from build123d import *

# Parameters (mm, degrees)
SKETCH1_R           = 2.5
BOSS_EXTRUDE1_DEPTH = 3
FILLET1_R           = 10
FILLET2_R           = 1
SKETCH2_R           = 1
CUT_EXTRUDE1_DEPTH  = 5


with BuildPart() as part:
    # Sketch1 → Boss-Extrude1 (new body)
    with BuildSketch(Plane.XY):
        with BuildLine():
            Line((-15.775199063, 25.595763214), (7.5, 42.17358061))
            Line((7.5, 42.17358061), (7.5, 47.084472248))
            Line((7.5, 47.084472248), (-21.353827366, 26.533263214))
            Line((-21.353827366, 26.533263214), (-10.092955814, 2.19356054))
            ThreePointArc((-10.092955814, 2.19356054), (-10.003238503, 2.060792281), (-9.876128914, 1.963223028))
            Line((-9.876128914, 1.963223028), (-7.240482475, 0.850547008))
            ThreePointArc((-7.240482475, 0.850547008), (-6.935224137, 0.406591519), (-7.210200963, -0.056730047))
            Line((-7.210200963, -0.056730047), (-9.9765648, -1.448728989))
            ThreePointArc((-9.9765648, -1.448728989), (-10.241411893, -1.996858986), (-9.780506444, -2.394548117))
            Line((-9.780506444, -2.394548117), (-6.921562347, -2.289102741))
            ThreePointArc((-6.921562347, -2.289102741), (-6.457280642, -2.56245531), (-6.510686125, -3.098577481))
            Line((-6.510686125, -3.098577481), (-8.429579039, -5.529272837))
            ThreePointArc((-8.429579039, -5.529272837), (-8.437962276, -6.137976541), (-7.852169389, -6.303618237))
            Line((-7.852169389, -6.303618237), (-5.305649232, -4.999810287))
            ThreePointArc((-5.305649232, -4.999810287), (-4.76934332, -5.051337921), (-4.591170105, -5.559799752))
            Line((-4.591170105, -5.559799752), (-5.303021449, -8.57371707))
            ThreePointArc((-5.303021449, -8.57371707), (-5.053369941, -9.128932885), (-4.45245808, -9.031488473))
            Line((-4.45245808, -9.031488473), (-2.695540082, -6.773631253))
            ThreePointArc((-2.695540082, -6.773631253), (-2.187705338, -6.593678477), (-1.811340311, -6.979202139))
            Line((-1.811340311, -6.979202139), (-1.182760229, -10.011580251))
            ThreePointArc((-1.182760229, -10.011580251), (-0.721854781, -10.409269381), (-0.21842547, -10.066998426))
            Line((-0.21842547, -10.066998426), (0.419671299, -7.278179214))
            ThreePointArc((0.419671299, -7.278179214), (0.803874553, -6.900466376), (1.307906448, -7.09081074))
            Line((1.307906448, -7.09081074), (3.159131837, -9.573429214))
            ThreePointArc((3.159131837, -9.573429214), (3.744924723, -9.73907091), (4.056536671, -9.216109658))
            Line((4.056536671, -9.216109658), (3.456242815, -6.418909742))
            ThreePointArc((3.456242815, -6.418909742), (3.644820872, -5.914214344), (4.182071907, -5.87371184))
            Line((4.182071907, -5.87371184), (6.909051797, -7.34136664))
            ThreePointArc((6.909051797, -7.34136664), (7.509963658, -7.243922228), (7.571367017, -6.638265473))
            Line((7.571367017, -6.638265473), (5.845168255, -4.356836553))
            ThreePointArc((5.845168255, -4.356836553), (5.802784524, -3.819730653), (6.272582224, -3.55597082))
            Line((6.272582224, -3.55597082), (9.364323053, -3.733646292))
            ThreePointArc((9.364323053, -3.733646292), (9.867752363, -3.391375337), (9.667441101, -2.816513723))
            Line((9.667441101, -2.816513723), (7.138800197, -1.478360048))
            ThreePointArc((7.138800197, -1.478360048), (6.87339673, -1.009488927), (7.187708321, -0.571896249))
            Line((7.187708321, -0.571896249), (10.064866009, 0.573701222))
            ThreePointArc((10.064866009, 0.573701222), (10.376477957, 1.096662475), (9.951987284, 1.533008835))
            Line((9.951987284, 1.533008835), (7.094732162, 1.677138107))
            ThreePointArc((7.094732162, 1.677138107), (6.656041435, 1.989915303), (6.75596982, 2.519342773))
            Line((6.75596982, 2.519342773), (8.879409827, 4.773546063))
            ThreePointArc((8.879409827, 4.773546063), (8.940813186, 5.379202818), (8.371686043, 5.595269411))
            Line((8.371686043, 5.595269411), (5.721221814, 4.5183667))
            ThreePointArc((5.721221814, 4.5183667), (5.191447637, 4.616440396), (5.058267794, 5.138496195))
            Line((5.058267794, 5.138496195), (6.030090531, 8.078902715))
            ThreePointArc((6.030090531, 8.078902715), (5.829779269, 8.653764329), (5.222661219, 8.609063642))
            Line((5.222661219, 8.609063642), (3.275643601, 6.512923743))
            ThreePointArc((3.275643601, 6.512923743), (2.754057404, 6.377916456), (2.41272516, 6.794775458))
            Line((2.41272516, 6.794775458), (2.050826183, 9.870398819))
            ThreePointArc((2.050826183, 9.870398819), (1.62633551, 10.306745179), (1.09499102, 10.009653423))
            Line((1.09499102, 10.009653423), (0.216260792, 7.287060309))
            ThreePointArc((0.216260792, 7.287060309), (-0.199400295, 6.944270302), (-0.684924592, 7.177819622))
            Line((-0.684924592, 7.177819622), (-2.312731053, 9.812335907))
            ThreePointArc((-2.312731053, 9.812335907), (-2.639135445, 10.039629661), (-3.028156876, 9.956776757))
            Line((-3.028156876, 9.956776757), (-4.095052713, 9.19687759))
            Line((-4.095052713, 9.19687759), (-15.775199063, 25.595763214))
        make_face()
        Circle(SKETCH1_R, mode=Mode.SUBTRACT)
    extrude(amount=BOSS_EXTRUDE1_DEPTH)

    # Fillet1
    fillet1_edges = [part.edges().sort_by_distance(p)[0] for p in [
        (-21.353827366, 26.533263214, 1.5),
        (-15.775199063, 25.595763214, 1.5),
    ]]
    fillet(fillet1_edges, radius=FILLET1_R)

    # Fillet2
    fillet2_edges = [part.edges().sort_by_distance(p)[0] for p in [
        (7.5, 47.084472248, 1.5),
        (7.5, 42.17358061, 1.5),
    ]]
    fillet(fillet2_edges, radius=FILLET2_R)

    # Sketch2 → Cut-Extrude1 (cut)
    with BuildSketch(Plane.XY.offset(3)):
        with Locations((-10.224511364, 10.975398278)):
            Circle(SKETCH2_R)
    extrude(amount=-CUT_EXTRUDE1_DEPTH, mode=Mode.SUBTRACT)


solid = part.part
Can you work these out from the model? Positions are in its coordinate system, mm. A direction names the side the tool comes from. Give positions to 0.01 mm unless a question says otherwise; leave off trailing zeros. Order: outer loops, then holes, each group sorted by start corner. A loop starts at its lowest first (then second) coordinate and runs counter-clockwise, first axis right, second up. Notation, with made-up numbers: M 72.5,15.5 L 100.5,15.5 A21 ccw 100.5,34.5 Z; hole C 23.25,23.25 d3. An arc over 180 degrees is marked long. Use one line per item in the form item = value.
Item 1: Will these pins go through, and if not, where does the flat tip stop? pin 1 Ø5 at (x, y) = (-9, 40.5) entering from -Z; pin 2 Ø0.7 at (y, z) = (44, 2) entering from +X; pin 3 Ø1 at (x, z) = (-2.5, 1) entering from -Y; pin 4 Ø1.5 at (y, z) = (40, 2.5) entering from +X.
Values follow:
pin_1 = through
pin_2 = 7.5
pin_3 = -7.16
pin_4 = 5.5
Item 2: If we section it at A-A, the plane z = 0.6: Count the separate pieces of the cut face and the enclosed holes in it, and give its area (3 significant figures).
Values follow:
separate_pieces = 1
enclosed_holes = 2
area = 505 mm^2
Item 3: Thinking about a two-plate mould opening in X: for faces 1 (the cylindrical face through (10.377, 1.088, 1.479)), 2 (the flat face through (-7.46, -4.3, 1.48)), 3 (the flat face through (-8.371, -2.343, 1.479)), which applies, pulls with the +X half, pulls with the -X half, needs draft (parallel to the pull), parting line crosses it, or undercut?
Values follow:
face_1 = pulls with the +X half
face_2 = pulls with the -X half
face_3 = undercut
Item 4: If I drill on line 1 along Y through (x, z) = (-9.5, 1.2); line 2 along X through (y, z) = (-8, 1.85); line 3 along Y through (x, z) = (8, 0.2), over which ranges is the centre line in solid material (lowest first)? Write a range as [from, to].
Values follow:
line_1 = [-2.38, -1.21], [1.8, 10.29], [11.66, 16.79], [29.67, 34.98]
line_2 = [-5.17, -3.65], [-1.6, 0.25], [1.99, 3.8]
line_3 = [-3.66, -1.93], [-0.25, 1.63], [3.84, 5.44]
Item 5: If we section it at B-B, the plane y = 21: Write out the boundary of the cut face in (x, z).
Values follow:
outline = M -18.55,0 L -11.57,0 L -11.57,3 L -18.55,3 Z
Item 6: For faces 4 (the flat face through (-8.57, -0.74, 1.48)), 5 (the flat face through (7.5, 44, 1)), 6 (the flat face through (8.421, -2.157, 1.479)), 7 (the flat face through (-3.59, -7.92, 1.48)), 8 (the flat face through (7.797, -3.644, 1.479)), which set-ups out of +Z, -Z, +X, -X, +Y, -Y let a thin tool reach every point of the face, with its end or its side?
Values follow:
face_4 = +Z, -Z, -X
face_5 = +Z, -Z, +X, +Y
face_6 = +Z, -Z, +X
face_7 = +Z, -Z, -Y
face_8 = +Z, -Z
